Print and shaded views of the part. All mm, measured from the part's lowest x, y and z. Round coordinates to 2 decimals unless told otherwise and drop trailing zeros. Order: outer loops, then holes, each group sorted by start corner. A loop starts at its lowest first (then second) coordinate and runs counter-clockwise, first axis right, second up. Notation, with made-up numbers: M 7.5,42.25 L 47.5,42.25 A18 ccw 47.5,63.25 Z; hole C -14,-36 d11. An arc over 180 degrees is marked long. Use CSV: the item, a comma, the result in double quotes.
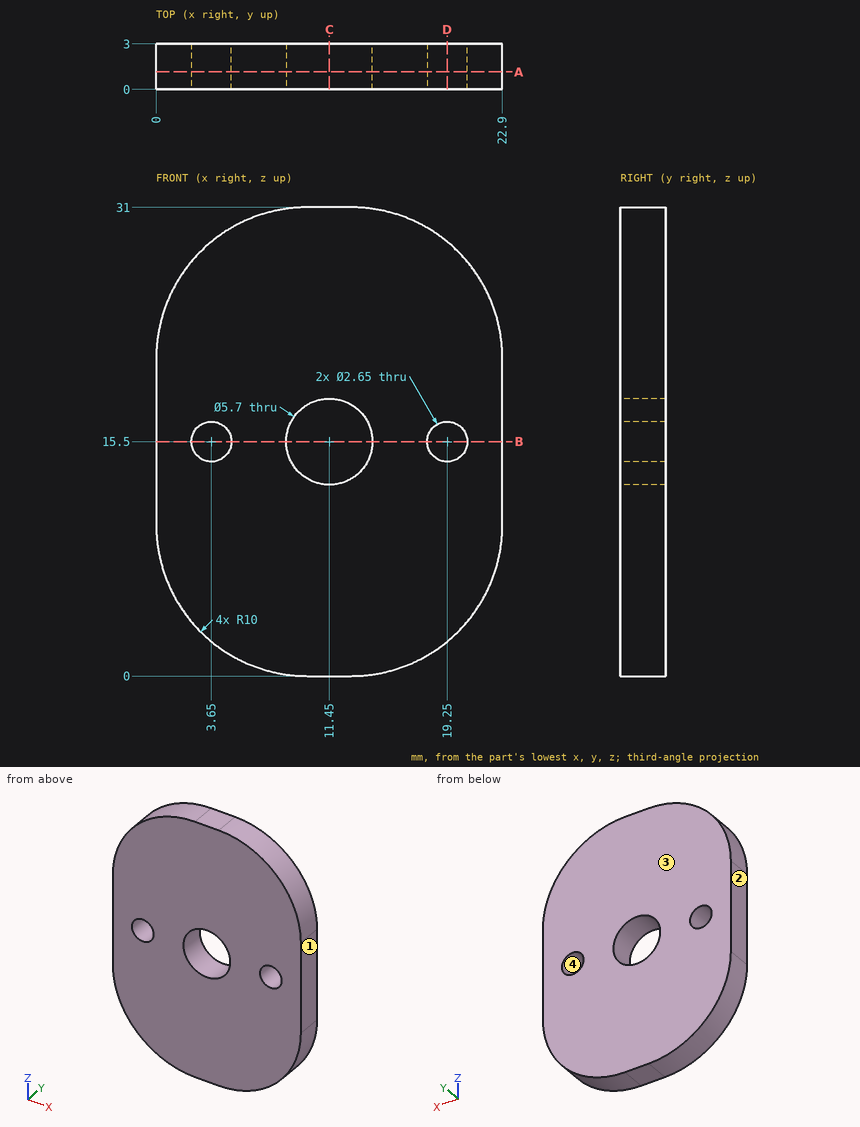
(1) Cut at B-B, the plane z = 15.5. Give the cut face in (x, y) (3 decimals), and give its area (3 significant figures).
Answer block:
outline,"M 0,0 L 2.325,0 L 2.325,3 L 0,3 Z; M 4.975,0 L 8.6,0 L 8.6,3 L 4.975,3 Z; M 14.3,0 L 17.925,0 L 17.925,3 L 14.3,3 Z; M 20.575,0 L 22.9,0 L 22.9,3 L 20.575,3 Z"
area,"35.7 mm²"
(2) Wall check: line 1 (X direction, y = 1.4, z = 15.5) (3 decimals); line 2 (Z direction, x = 11.45, y = 1); line 3 (X direction, y = 1.9, z = 18). Give the ranges that are in metal, low to high. Write a range as from..to.
Answer block:
line 1,"x = 0..2.325, 4.975..8.6, 14.3..17.925, 20.575..22.9"
line 2,"z = 0..12.65, 18.35..31"
line 3,"x = 0..10.08, 12.82..22.9"
(3) Cut at C-C, the plane x = 11.45. Give the cut face in (y, z), and give its area (3 significant figures).
Answer block:
outline,"M 0,0 L 3,0 L 3,12.65 L 0,12.65 Z; M 0,18.35 L 3,18.35 L 3,31 L 0,31 Z"
area,"75.9 mm²"
(4) Cut at A-A, the plane y = 1.15. Give the cut face in (x, z) (3 decimals), and give its area (3 significant figures).
Answer block:
outline,"M 0,10 A10 ccw 10,0 L 12.9,0 A10 ccw 22.9,10 L 22.9,21 A10 ccw 12.9,31 L 10,31 A10 ccw 0,21 Z; hole C 3.65,15.5 d2.65; hole C 11.45,15.5 d5.7; hole C 19.25,15.5 d2.65"
area,"588 mm²"
(5) Two-plate mould, pull along X, no slides. Class the marked faces 1, 2, 3 and 4: released by +X, released by -X, zero draft, split by the parting line, or undercut.
Answer block:
face 1,"released by +X"
face 2,"released by -X"
face 3,"zero draft"
face 4,"undercut"
(6) Drop flat-ended pins along their axis: pin 1 (2 mm diameter, centred on x = 19.25, z = 15.5, fed in from +Y); pin 2 (1.5 mm diameter, centred on y = 2.5, z = 5.5, fed in from +X). Give the stop position or say it passes through.
Answer block:
pin 1,"passes through"
pin 2,"stops at x = 22.17"
(7) Cut at D-D, the plane x = 19.25. Give the cut face in (y, z) (3 decimals).
Answer block:
outline,"M 0,2.275 L 3,2.275 L 3,14.175 L 0,14.175 Z; M 0,16.825 L 3,16.825 L 3,28.725 L 0,28.725 Z"
